Verification items for the finished model (mm, model axes). A direction names the side the tool comes from. Give positions to 0.01 mm unless a question says otherwise; leave off trailing zeros. Write each loop counter-clockwise with the first axis right and the second up, starting at its lowest first coordinate (ties: lowest second). Pieces come first, ordered by that corner, then holes.
Autodesk Inventor part; units mm, degrees
ref_plane "YZ Plane" through (0, 0, 0) normal (1, 0, 0) x (0, 1, 0)
ref_plane "XZ Plane" through (0, 0, 0) normal (0, 1, 0) x (-1, 0, 0)
ref_plane "XY Plane" through (0, 0, 0) normal (0, 0, 1) x (1, 0, 0)
sketch "Sketch1" plane through (0, 0, 0) normal (0, 0, 1) x (1, 0, 0)
  line L0 (0.5, 0) -> (19.5, 0)
  line L1 (19.5, 14) -> (0.5, 14)
  line L2 (-0.5, 12.795) -> (-1.405, 12.795)
  line L3 (-1.405, 1.205) -> (-0.5, 1.205)
  line L4 (20.5, 12.795) -> (21.405, 12.795)
  line L5 (21.405, 1.205) -> (20.5, 1.205)
  line L6 (0, 13.5) -> (0, 13.295)
  line L7 (0, 0.705) -> (0, 0.5)
  line L8 (20, 0.5) -> (20, 0.705)
  line L9 (20, 13.295) -> (20, 13.5)
  circle A0 centre (-3.6, 7) radius 2
  circle A1 centre (23.6, 7) radius 2
  line L10 (3.975, 12.525) -> (16.025, 12.525)
  line L11 (16.025, 12.525) -> (16.025, 1.475)
  line L12 (16.025, 1.475) -> (3.975, 1.475)
  line L13 (3.975, 1.475) -> (3.975, 12.525)
  arc A2 (0.5, 14) -> (0, 13.5) centre (0.5, 13.5) ccw
  arc A3 (-0.5, 12.795) -> (0, 13.295) centre (-0.5, 13.295) ccw
  arc A4 (20, 13.5) -> (19.5, 14) centre (19.5, 13.5) ccw
  arc A5 (20, 13.295) -> (20.5, 12.795) centre (20.5, 13.295) ccw
  arc A6 (20.5, 1.205) -> (20, 0.705) centre (20.5, 0.705) ccw
  arc A7 (19.5, 0) -> (20, 0.5) centre (19.5, 0.5) ccw
  arc A8 (0, 0.5) -> (0.5, 0) centre (0.5, 0.5) ccw
  arc A9 (0, 0.705) -> (-0.5, 1.205) centre (-0.5, 0.705) ccw
  line L14 (10, 15.3107) -> (10, 19.4603)
  arc A10 (-1.405, 12.795) -> (-1.405, 1.205) centre (-1.405, 7) ccw
  arc A11 (21.405, 1.205) -> (21.405, 12.795) centre (21.405, 7) ccw
  line L15 (-7.2, 7) -> (-7.2, 15.3107)
  point P0 (0, 0)
  point P1 (20, 14)
  point P2 (20, 0)
  point P3 (0, 14)
  point P4 (0, 12.795)
  point P5 (0, 1.205)
  point P6 (20, 12.795)
  point P7 (20, 1.205)
  dimension "d0" = 11.59
  dimension "d1" = 1.205
  dimension "d2" = 4
  dimension "width" = 20
  dimension "height" = 14
  dimension "d7" = 12.05
  dimension "d8" = 11.05
  dimension "d9" = 3.975
  dimension "d10" = 1.475
  dimension "d13" = 0.5
  dimension "d31" = 27.2
  dimension "d32" = 13.6
  dimension "d33" = 10
  dimension "d34" = 34.4
  dimension "d35" = 17.2
extrude "Extrusion1" add sketch "Sketch1" against normal blind 10
sketch "Sketch3" plane through (0, 0, -10) normal (0, 0, -1) x (-1, 0, 0)
  line L0 (-19.5, 14) -> (-0.5, 14)
  line L1 (0, 13.5) -> (0, 0.5)
  line L2 (-0.5, 0) -> (-19.5, 0)
  line L3 (-20, 0.5) -> (-20, 13.5)
  line L4 (-0.5, 0) -> (-19.5, 0)
  line L5 (0, 0.5) -> (0, 0.705)
  arc A0 (0, 13.5) -> (-0.5, 14) centre (-0.5, 13.5) ccw
  arc A1 (-0.5, 0) -> (0, 0.5) centre (-0.5, 0.5) ccw
  arc A2 (-20, 0.5) -> (-19.5, 0) centre (-19.5, 0.5) ccw
  arc A3 (-19.5, 14) -> (-20, 13.5) centre (-19.5, 13.5) ccw
  point P0 (0, 0)
  point P1 (-20, 14)
  point P2 (0, 0)
  point P3 (0, 14)
  point P4 (-20, 0)
  dimension "d14" = 20
  dimension "d15" = 14
  dimension "d16" = 0
  dimension "d17" = 0
  dimension "d20" = 0.5
extrude "Extrusion2" add sketch "Sketch3" along normal blind 19.32
sketch "Sketch6" plane through (0.5, 14, 0) normal (0, 1, 0) x (1, 0, 0)
  line L0 (-0.5, 0) -> (-0.5, 29.32)
  line L1 (-0.5, 29.32) -> (-0.5, 26.32)
  line L2 (-0.5, 29.32) -> (2.5, 29.32)
  arc A0 (2.5, 29.32) -> (-0.5, 26.32) centre (2.5, 26.32) ccw
  line L3 (19.5, 0) -> (19.5, 29.32)
  line L4 (19.5, 29.32) -> (19.5, 26.32)
  line L5 (19.5, 29.32) -> (16.5, 29.32)
  line L6 (0, 29.32) -> (19, 29.32)
  arc A1 (19.5, 26.32) -> (16.5, 29.32) centre (16.5, 26.32) ccw
  dimension "d36" = 3
extrude "Extrusion4" cut sketch "Sketch6" against normal through all
fillet "Fillet2" radius 0.5 10 edges at (18.4186, 14, -28.9634) (19.8751, 13.8307, -27.1768) (1.5814, 14, -28.9634) (0.1247, 13.8304, -27.176) (10, 14, -29.32) (1.5814, 0, -28.9634) (0.1249, 0.1694, -27.1767) (18.4186, 0, -28.9634) (19.8753, 0.1696, -27.176) (10, 0, -29.32)
sketch "Sketch7" plane through (0, 0, -29.32) normal (0, 0, -1) x (-1, 0, 0)
  circle A0 centre (-10, 7) radius 4.625
  line L0 (-3, 14) -> (-17, 14)
  line L1 (-20, 0.5) -> (-20, 13.5)
  point P0 (0, 0)
  dimension "d40" = 9.25
  dimension "d41" = 7
  dimension "d42" = 10
extrude "Extrusion5" add sketch "Sketch7" along normal blind 5
equation "\"d1\" = -0.5 * d0 + 0.5 * height"
equation "\"d9\" = -0.5 * d7 + 0.5 * width"
equation "\"d10\" = -0.5 * d8 + 0.5 * height"
equation "\"d32\" = 0.5 * d31"
equation "\"d33\" = 0.5 * width"
equation "\"d35\" = 0.5 * d34"
equation "\"d16\" = -0.5 * d15 + 0.5 * height"
equation "\"d17\" = -0.5 * d14 + 0.5 * width"
equation "\"d41\" = 0.5 * height"
equation "\"d42\" = 0.5 * width"
properties part number "panel-mount"
Item 1: Scan lines: line 1 along Y through (x, z) = (14.5, -2) (3 decimals); line 2 along X through (y, z) = (5.25, -6) (3 decimals); line 3 along X through (y, z) = (12.25, -12). Record each from-to range of solid material in increasing order.
Answer key:
line 1: y = 0 to 1.475, 12.525 to 14
line 2: x = -6.929 to -4.568, -2.632 to 3.975, 16.025 to 22.632, 24.568 to 26.929
line 3: x = 0 to 20
Item 2: Depth check by flat-ended pin: pin 1 (4 mm diameter, centred on y = 9, z = -15.5, fed in from +X); pin 2 (3.5 mm diameter, centred on x = 8.5, y = 9, fed in from +Z); pin 3 (4 mm diameter, centred on y = 9, z = -15.5, fed in from -X). Enter the tip coordinate at first touch or a pass-through.
Answer key:
pin 1: stops at x = 20
pin 2: stops at z = -10
pin 3: stops at x = 0
Item 3: Sectioned sample at A-A on y = 7. Record the cut outline in (x, z) (3 decimals), then the cut area to 3 significant figures.
Answer key:
outline: (-7.2, -10) - (-5.6, -10) - (-5.6, 0) - (-7.2, 0) - close; (-1.6, -10) - (0, -10) - (0, -26.32) arc R3 ccw to (3, -29.32) - (5.375, -29.32) - (5.375, -34.32) - (14.625, -34.32) - (14.625, -29.32) - (17, -29.32) arc R3 ccw to (20, -26.32) - (20, -10) - (21.6, -10) - (21.6, 0) - (16.025, 0) - (16.025, -10) - (3.975, -10) - (3.975, 0) - (-1.6, 0) - close; (25.6, -10) - (27.2, -10) - (27.2, 0) - (25.6, 0) - close
area: 572 mm2
Item 4: Set-up check for faces 4 (the face through (21, 7, -10)), 5 (the face through (15, 7, -29.32)), 6 (the face through (3.975, 7, -5)), 7 (the face through (21, 1.205, -5)), 8 (the face through (-1, 7, -10)): record each of +Z, -Z, +X, -X, +Y, -Y from which the full face is reachable in a straight line by a thin tool's end or side.
Answer key:
face 4: -Z, +X, +Y, -Y
face 5: -Z
face 6: +Z
face 7: +Z, -Z, +X, -Y
face 8: -Z, -X, +Y, -Y
Item 5: Sectioned sample at B-B on x = 23.6. Record the cut outline in (y, z).
Answer key:
outline: (1.64, -10) - (5, -10) - (5, 0) - (1.64, 0) - close; (9, -10) - (12.36, -10) - (12.36, 0) - (9, 0) - close
Item 6: Sectioned sample at D-D on y = 4.5. Record the cut outline in (x, z) (3 decimals).
Answer key:
outline: (-6.633, -10) - (0, -10) - (0, -26.32) arc R3 ccw to (3, -29.32) - (6.109, -29.32) - (6.109, -34.32) - (13.891, -34.32) - (13.891, -29.32) - (17, -29.32) arc R3 ccw to (20, -26.32) - (20, -10) - (26.633, -10) - (26.633, 0) - (16.025, 0) - (16.025, -10) - (3.975, -10) - (3.975, 0) - (-6.633, 0) - close
Item 7: Sectioned sample at C-C on x = 10. Record the cut outline in (y, z) (3 decimals), then the cut area to 3 significant figures.
Answer key:
outline: (0, -28.82) arc R0.5 ccw to (0.5, -29.32) - (2.375, -29.32) - (2.375, -34.32) - (11.625, -34.32) - (11.625, -29.32) - (13.5, -29.32) arc R0.5 ccw to (14, -28.82) - (14, 0) - (12.525, 0) - (12.525, -10) - (1.475, -10) - (1.475, 0) - (0, 0) - close
area: 346 mm2
Item 8: Release check for a two-part mould opening along Y. For faces 1 (the face through (10, 0, -14)), 2 (the face through (10, 12.525, -5)), 3 (the face through (-7.2, 7.1, -4.9)) record: released by +Y, released by -Y, zero draft, split by the parting line, or undercut.
Answer key:
face 1: released by -Y
face 2: undercut
face 3: split by the parting line
